The model under review builds one solid part; all positions refer to its coordinate system, in mm. A direction names the side the tool comes from. Coordinates: 2 decimals unless noted, no trailing zeros. Order: outer loops, then holes, each group sorted by start corner. A loop starts at its lowest first (then second) coordinate and runs counter-clockwise, first axis right, second up. Notation, with made-up numbers: M 45.5,7 L 70.5,7 A7 cw 70.5,18 Z; hole C 10.25,-36.75 d8. An arc over 180 degrees is marked long. Answer in a Markdown table with one row per item.
from build123d import *

# Parameters (mm, degrees)
SALIENTE_EXTRUIR1_DEPTH      = 25
SALIENTE_EXTRUIR1_DEPTH_BACK = 25
CROQUIS2_R                   = 22.5
CORTAR_EXTRUIR1_REACH        = 122.147
CORTAR_EXTRUIR1_END_RADIUS   = 22.5
CROQUIS3_R                   = 6.164928148


with BuildPart() as part:
    # Croquis2 → Saliente-Extruir1 (new, two sides: drawn at the far end of the back side and taken through both)
    with BuildSketch(Plane.XY.offset(-SALIENTE_EXTRUIR1_DEPTH_BACK)):
        with BuildLine():
            Line((-40, 53), (-40, 93))
            Line((-40, 93), (-30, 93))
            Line((-30, 93), (-6.164928148, 73))
            Line((-6.164928148, 73), (6.164928148, 73))
            Line((6.164928148, 73), (30, 93))
            Line((30, 93), (40, 93))
            Line((40, 93), (40, 53))
            ThreePointArc((40, 53), (27.282813289, 40.082394099), (30.225762041, 22.19579485))
            ThreePointArc((30.225762041, 22.19579485), (0, -37.5), (-30.225762041, 22.19579485))
            ThreePointArc((-30.225762041, 22.19579485), (-27.282813289, 40.082394099), (-40, 53))
        make_face()
        Circle(CROQUIS2_R, mode=Mode.SUBTRACT)
    extrude(amount=SALIENTE_EXTRUIR1_DEPTH + SALIENTE_EXTRUIR1_DEPTH_BACK)

    # Cortar-Extruir1: up to this cylinder (the profile starts outside it)
    cortar_extruir1_end = Plane(origin=(0, 0, 0), z_dir=(0, 0, 1)) * Cylinder(CORTAR_EXTRUIR1_END_RADIUS, 290.294, mode=Mode.PRIVATE)
    # Croquis3 → Cortar-Extruir1 (cut, up to the surface)
    with BuildSketch(Plane(origin=(0, 73, 0), x_dir=(1, 0, 0), z_dir=(0, 1, 0)), mode=Mode.PRIVATE) as cortar_extruir1_sk1:
        with Locations(Location((0, 0, 0), (0, 0, 270))):
            Circle(CROQUIS3_R)
    cortar_extruir1_tool1 = extrude(cortar_extruir1_sk1.sketch, amount=-CORTAR_EXTRUIR1_REACH, mode=Mode.PRIVATE) - cortar_extruir1_end
    add(cortar_extruir1_tool1.solids().sort_by_distance((0, 73, 0))[0], mode=Mode.SUBTRACT)


solid = part.part
(1) The part is to be moulded in two halves that separate along X. For faces 1 (the cylindrical face through (1.157, -37.482, -0.35)), 2 (the flat face through (-35, 93, 0)), 3 (the flat face through (0, 73, 15)), 4 (the cylindrical face through (27.364, 40.333, -0.35)), say which applies: +X half, -X half, draft (parallel to the pull), parting line (faces both ways), or undercut.
Report:
| item | result |
|---|---|
| face 1 | parting line |
| face 2 | draft |
| face 3 | undercut |
| face 4 | +X half |
(2) Take a section at D-D (z = 12). Write out the cut boundary in (x, y).
Report:
| item | result |
|---|---|
| outline | M -40,53 A20 cw -30.23,22.2 A37.5 ccw long 30.23,22.2 A20 cw 40,53 L 40,93 L 30,93 L 6.16,73 L -6.16,73 L -30,93 L -40,93 Z; hole C 0,0 d45 |
(3) Take a section at A-A (y = 0). Write out the cut boundary in (x, z), then the cut area to 3 significant figures.
Report:
| item | result |
|---|---|
| outline | M -37.5,-25 L -22.5,-25 L -22.5,25 L -37.5,25 Z; M 22.5,-25 L 37.5,-25 L 37.5,25 L 22.5,25 Z |
| area | 1,500 mm^2 |
(4) Take a section at B-B (x = 0). Write out the cut boundary in (y, z).
Report:
| item | result |
|---|---|
| outline | M -37.5,-25 L -22.5,-25 L -22.5,25 L -37.5,25 Z; M 22.5,-25 L 73,-25 L 73,-6.16 L 22.5,-6.16 Z; M 22.5,6.16 L 73,6.16 L 73,25 L 22.5,25 Z |
(5) To check wall thickness, follow line 1 (X direction, y = 58, z = 0); line 2 (Z direction, x = 0, y = 41); line 3 (Y direction, x = 0, z = 13). State the ranges of each line that lie inside material, in increasing order. Write a range as [from, to].
Report:
| item | result |
|---|---|
| line 1 | [-40, -6.16], [6.16, 40] |
| line 2 | [-25, -6.16], [6.16, 25] |
| line 3 | [-37.5, -22.5], [22.5, 73] |
(6) Machinability: for faces 5 (the flat face through (1, 29, 25)), 6 (the flat face through (0, 73, -15)), 7 (the cylindrical face through (-3.751, 47.678, -4.892)), which of the approach directions +Z, -Z, +X, -X, +Y, -Y give a long, thin tool a straight path to every point of the face, cutting with its end or side? Answer none if there is none.
Report:
| item | result |
|---|---|
| face 5 | +Z, +X, -X, +Y, -Y |
| face 6 | +Z, -Z, +Y |
| face 7 | +Y |
(7) Insertion check: P1, Ø10, axis at x = 0, z = 0, coming from the -Y side; P2, Ø1, axis at y = 37, z = 11, coming from the +X side; P3, Ø6, axis at x = -3, z = -10.5, coming from the +Y side. Each pin has a flat end and moves straight along its axis. Give the tip position at first contact, or say it passes through.
Report:
| item | result |
|---|---|
| P1 | y = -37.5 |
| P2 | x = 26.65 |
| P3 | y = 73 |
(8) Take a section at C-C (x = -13). Write out the cut boundary in (y, z).
Report:
| item | result |
|---|---|
| outline | M -35.17,-25 L -18.36,-25 L -18.36,25 L -35.17,25 Z; M 18.36,-25 L 78.74,-25 L 78.74,25 L 18.36,25 Z |
